Source: CAD feature listing. Evaluate the final solid. Frame: model axes, mm. Face numbers are marked on the shaded views. A direction names the side the tool comes from. Round coordinates to 2 decimals unless told otherwise and drop trailing zeros. Write each loop counter-clockwise with the first axis right and the second up, starting at its lowest first coordinate (ties: lowest second). Pieces come first, ordered by that corner, then holes. Notation, with made-up numbers: M 76,88 L 82,88 A22 cw 82,115 Z; hole C 71.5,11 d1. An arc over 180 degrees is marked long. Put each result on its own line as item: value. Start each with the question number.
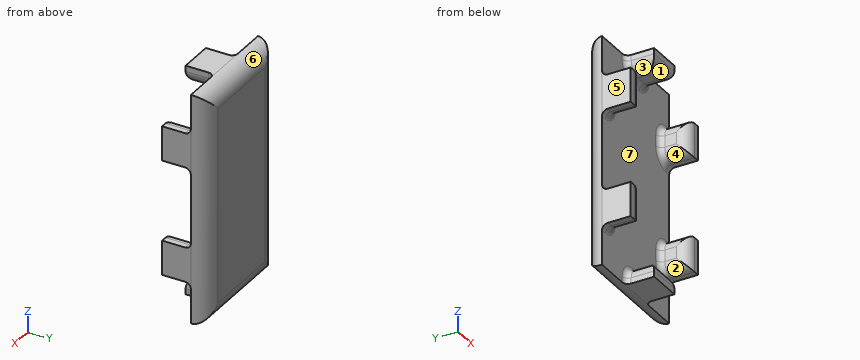
```python
from build123d import *

# Parameters (mm, degrees)
ESBO_O1_W                = 20
ESBO_O1_H                = 40
RESSALTO_EXTRUS_O1_DEPTH = 3
FILETE1_R                = 3
ESBO_O2_W                = 6
ESBO_O2_H                = 3
ESBO_O2_W_2              = 3
ESBO_O2_H_2              = 6
RESSALTO_EXTRUS_O2_DEPTH = 5
FILETE2_R                = 2
FILETE3_R                = 1


with BuildPart() as part:
    # Esboço1 → Ressalto-extrusão1 (new body)
    with BuildSketch(Plane(origin=(0, 0, 0), x_dir=(1, 0, 0), z_dir=(0, 1, 0))):
        with Locations((10, 20)):
            Rectangle(ESBO_O1_W, ESBO_O1_H)
    extrude(amount=RESSALTO_EXTRUS_O1_DEPTH)

    # Filete1
    filete1_edges = [part.edges().sort_by_distance(p)[0] for p in [
        (10, 3, -40),
        (20, 3, -20),
        (10, 3, 0),
        (0, 3, -20),
    ]]
    fillet(filete1_edges, radius=FILETE1_R - 0.0001)  # a hair under: the kernel refuses the full size

    # Esboço2 → Ressalto-extrusão2 (add)
    with BuildSketch(Plane.XZ):
        with Locations((10, -1.5)):
            Rectangle(ESBO_O2_W, ESBO_O2_H)
        with Locations((10, -38.5)):
            Rectangle(ESBO_O2_W, ESBO_O2_H)
        with Locations((1.5, -30)):
            Rectangle(ESBO_O2_W_2, ESBO_O2_H_2)
        with Locations((18.5, -10)):
            Rectangle(ESBO_O2_W_2, ESBO_O2_H_2)
        with Locations((18.5, -30)):
            Rectangle(ESBO_O2_W_2, ESBO_O2_H_2)
        with Locations((1.5, -10)):
            Rectangle(ESBO_O2_W_2, ESBO_O2_H_2)
    extrude(amount=RESSALTO_EXTRUS_O2_DEPTH)

    # Filete2
    filete2_edges = [part.edges().sort_by_distance(p)[0] for p in [
        (13, -2.5, -3),
        (7, -2.5, -3),
        (10, -5, -3),
        (7, -2.5, -37),
        (13, -2.5, -37),
        (10, -5, -37),
        (17, -2.5, -7),
        (17, -2.5, -13),
        (17, -5, -10),
        (17, -2.5, -27),
        (17, -2.5, -33),
        (17, -5, -30),
        (3, -2.5, -33),
        (3, -2.5, -27),
        (3, -5, -30),
        (3, -2.5, -13),
        (3, -2.5, -7),
        (3, -5, -10),
    ]]
    fillet(filete2_edges, radius=FILETE2_R)

    # Filete3
    filete3_edges = [part.edges().sort_by_distance(p)[0] for p in [
        (3, 0, -30),
        (0.5, 0, -27),
        (19.5, 0, -33),
        (17, 0, -30),
        (19.5, 0, -13),
        (17, 0, -10),
        (10, 0, -3),
        (13, 0, -0.5),
        (3, 0, -10),
        (0.5, 0, -7),
        (7.585786438, 0, -37.585786438),
        (12.414213562, 0, -37.585786438),
        (2.414213562, 0, -32.414213562),
        (2.414213562, 0, -27.585786438),
        (17.585786438, 0, -32.414213562),
        (17.585786438, 0, -27.585786438),
        (17.585786438, 0, -12.414213562),
        (17.585786438, 0, -7.585786438),
        (7.585786438, 0, -2.414213562),
        (12.414213562, 0, -2.414213562),
        (2.414213562, 0, -12.414213562),
        (2.414213562, 0, -7.585786438),
        (7, 0, -0.5),
        (13, 0, -39.5),
        (19.5, 0, -7),
        (19.5, 0, -27),
        (0.5, 0, -33),
        (0.5, 0, -13),
        (7, 0, -39.5),
        (10, 0, -37),
    ]]
    fillet(filete3_edges, radius=FILETE3_R)


solid = part.part
```
(1) Ray query, line 1 along X through (y, z) = (-3, -11); line 2 along Y through (x, z) = (14.5, -30.5); line 3 along Z through (x, y) = (10.75, -1.25). Return the intervals inside material, ascending.
(2) Access query for the marked faces 1, 2, 3 and 4. Directions: +Z, -Z, +X, -X, +Y, -Y. A direction counts if a zero-diameter tool reaches every point of the face in a straight line with its end or side. Return the directions, or none.
(3) Section query B-B (x = 10). Return loops of the section in (y, z), and give its area (3 significant figures).
(4) Section query C-C (y = -4). Count the separate pieces of the cut face and the enclosed holes in it, and give its area (3 significant figures).
(5) Pull-direction query (X, two-part tool) for the marked faces 5, 6 and 7; classes: +X half, -X half, draft (parallel to the pull), parting line (faces both ways), or undercut.
(6) Section query A-A (z = -10.5). Return loops of the section in (x, y).
(7) Contact query for flat-ended pins moving along their axis: P1, Ø0.8, axis at x = 19.5, y = -3, coming from the +Z side; P2, Ø1.1, axis at x = 0.5, y = -3, coming from the -Z side; P3, Ø1.1, axis at y = -2.5, z = -0.5, coming from the +X side. Output: stop coordinate, or through.
Entries:
1. line 1: 0 to 3, 17 to 20
1. line 2: 0 to 3
1. line 3: -40 to -37, -3 to 0
2. face 1: +X, -X, -Y
2. face 2: -Z, -Y
2. face 3: -X, -Y
2. face 4: -Y
3. outline: M -5,-40 L 0,-40 A3 ccw 3,-37 L 3,-3 A3 ccw 0,0 L -5,0 L -5,-1 A2 ccw -3,-3 L -1,-3 A1 cw 0,-4 L 0,-36 A1 cw -1,-37 L -3,-37 A2 ccw -5,-39 Z
3. area: 145 mm2
4. separate pieces: 6
4. enclosed holes: 0
4. area: 92.3 mm2
5. face 5: -X half
5. face 6: draft
5. face 7: undercut
6. outline: M 0,-5 L 1,-5 A2 ccw 3,-3 L 3,-1 A1 cw 4,0 L 16,0 A1 cw 17,-1 L 17,-3 A2 ccw 19,-5 L 20,-5 L 20,0 A3 ccw 17,3 L 3,3 A3 ccw 0,0 Z
7. P1: z = -7
7. P2: z = -33
7. P3: x = 13
